Source: CAD feature listing. Evaluate the final solid. Frame: model axes, mm. A direction names the side the tool comes from. Round coordinates to 2 decimals unless told otherwise and drop trailing zeros. Loops run counter-clockwise (first coordinate to the right, second up) from the corner with the lowest first, then second, coordinate; pieces in that order, holes last.
(1) First-contact query: pin 1 Ø0.7 at (x, z) = (4, 17) entering from -Y; pin 2 Ø3 at (x, z) = (-1.5, -27) entering from -Y; pin 3 Ø1.7 at (x, z) = (0.5, -16) entering from -Y; pin 4 Ø1.5 at (x, y) = (4, -7) entering from -Z. Flat tips, straight axial feed; report the tip coordinate or a pass-through.
(2) Material intervals for probe 1 along X at (y, z) = (7.5, -33.5); probe 2 along Y at (x, z) = (-4, -61.5); probe 3 along X at (y, z) = (3.75, -56.5), sorted ascending.
(3) Set-up query: faces 1 (the flat face through (10, -7, 1)), 2 (the flat face through (-3.901, 0, 1)), 3 (the flat face through (0, 3.901, 1)). Return all of +Z, -Z, +X, -X, +Y, -Y with unobstructed straight access to the full face (end or side cutting, diameter ignored); none if empty.
(4) Section A-A, the plane x = 1. Return the cut outline in (y, z), plus the area to 3 significant figures.
(5) Mould query, pull axis Y, two halves, no side actions, for faces 4 (the flat face through (3.901, 0, 1)), 5 (the flat face through (0, -3.901, 1)), 6 (the flat face through (0, 0, -100)). Classes: pulls with the +Y half, pulls with the -Y half, needs draft (parallel to the pull), parting line crosses it, or undercut.
```python
from build123d import *

# Parameters (mm, degrees)
PAD_DEPTH            = 100
PAD_MIRRORED_2_DEPTH = 100
POLARPATTERN_COUNT   = 4


with BuildPart() as part:
    # Sketch → Pad (new body, symmetric)
    with BuildSketch(Plane.XY):
        Polygon((10, 10), (4.9, 10), (3.1, 8.2), (5.49934, 8.2), (5.49934, 6.56), (2.84, 3.90066), (0, 3.90066), (0, 0), align=None)
    pad = extrude(amount=PAD_DEPTH, both=True)

    # Sketch Mirrored 2 → Pad Mirrored 2 (add, symmetric)
    with BuildSketch(Plane(origin=(0, 0, 0), x_dir=(-1, 0, 0), z_dir=(0, 0, -1))):
        Polygon((10, 10), (4.9, 10), (3.1, 8.2), (5.49934, 8.2), (5.49934, 6.56), (2.84, 3.90066), (0, 3.90066), (0, 0), align=None)
    pad_mirrored_2 = extrude(amount=-PAD_MIRRORED_2_DEPTH, both=True)

    # PolarPattern: Pad, Pad Mirrored 2 ×4 about axis
    polarpattern_axis = Axis((0, 0, 0), (0, 0, 1))
    for i in range(1, POLARPATTERN_COUNT):
        add(pad.rotate(polarpattern_axis, i * 360 / POLARPATTERN_COUNT))
        add(pad_mirrored_2.rotate(polarpattern_axis, i * 360 / POLARPATTERN_COUNT))


solid = part.part
```
Output values:
1. pin 1: stops at y = -9.45
1. pin 2: stops at y = -4.06
1. pin 3: stops at y = -3.9
1. pin 4: passes through
2. probe 1: x = -10 to -5.5, 5.5 to 10
2. probe 2: y = -9.1 to -8.2, -5.06 to -2.94, 2.94 to 5.06, 8.2 to 9.1
2. probe 3: x = -8.85 to -8.2, -4.81 to 4.81, 8.2 to 8.85
3. face 1: +Z, -Z, +X, +Y, -Y
3. face 2: +Z, -Z, -X
3. face 3: +Z, -Z, +Y
4. outline: (-3.9, -100) - (3.9, -100) - (3.9, 100) - (-3.9, 100) - close
4. area: 1,560 mm2
5. face 4: undercut
5. face 5: pulls with the -Y half
5. face 6: needs draft
